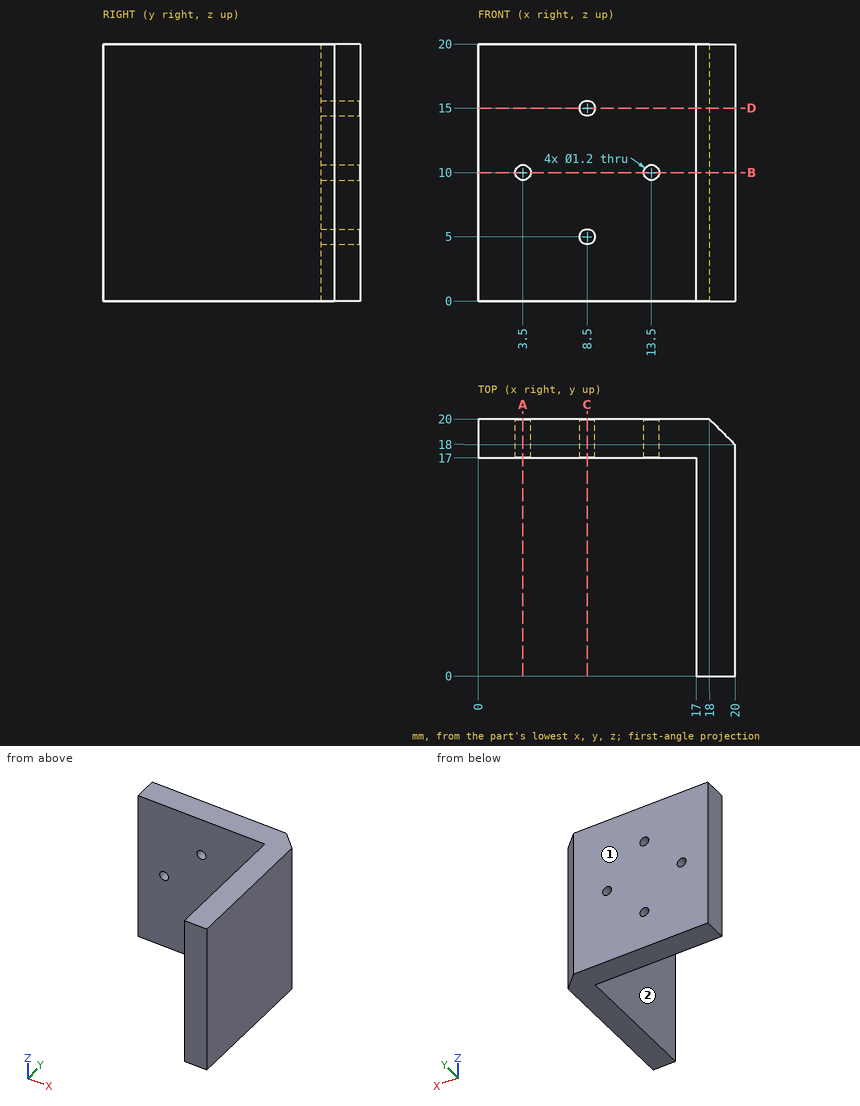
Study the drawing (mm; zero at the part's minimum x, y, z) and answer. A direction names the side the tool comes from. Round coordinates to 2 decimals unless told otherwise and drop trailing zeros. Write each loop counter-clockwise with the first axis right and the second up, starting at its lowest first coordinate (ties: lowest second). Pieces come first, ordered by that corner, then holes.
Q1. Find section B-B on z = 10. Determine the outline of the cut face in (x, y).
Values:
outline: (0, 17) - (2.9, 17) - (2.9, 20) - (0, 20) - close; (4.1, 17) - (12.9, 17) - (12.9, 20) - (4.1, 20) - close; (14.1, 17) - (17, 17) - (17, 0) - (20, 0) - (20, 18) - (18, 20) - (14.1, 20) - close
Q2. A tool of negligible diameter and unlimited length cuts with its end or side. For the marked faces 1 and 2, from which of +Z, -Z, +X, -X, +Y, -Y can it reach the whole face along a straight path? Write none if from no direction.
Values:
face 1: +Z, -Z, +X, -X, +Y
face 2: +Z, -Z, -X, -Y
Q3. Find section C-C on x = 8.5. Determine the outline of the cut face in (y, z).
Values:
outline: (17, 0) - (20, 0) - (20, 4.4) - (17, 4.4) - close; (17, 5.6) - (20, 5.6) - (20, 14.4) - (17, 14.4) - close; (17, 15.6) - (20, 15.6) - (20, 20) - (17, 20) - close
Q4. Flat-ended cylindrical pins translate along their axes: P1, Ø1.4, axis at x = 8.5, z = 15, coming from the -Y side; P2, Ø0.7, axis at x = 3.5, z = 10, coming from the -Y side; P3, Ø5, axis at y = 4.5, z = 5.5, coming from the -X side. Find the tip coordinate at first contact, or state that the pin passes through.
Values:
P1: stops at y = 17
P2: passes through
P3: stops at x = 17
Q5. Straight lines are drawn through the part: line 1 (Z direction, x = 13.5, y = 18.3); line 2 (X direction, y = 17.6, z = 5); line 3 (Y direction, x = 7.5, z = 12.75). For each, find the intervals that lie inside material, in ascending order.
Values:
line 1: z = 0 to 9.4, 10.6 to 20
line 2: x = 0 to 7.9, 9.1 to 20
line 3: y = 17 to 20
Q6. Find section A-A on x = 3.5. Determine the outline of the cut face in (y, z), and give its area (3 significant figures).
Values:
outline: (17, 0) - (20, 0) - (20, 9.4) - (17, 9.4) - close; (17, 10.6) - (20, 10.6) - (20, 20) - (17, 20) - close
area: 56.4 mm2
Q7. Find section D-D on z = 15. Determine the outline of the cut face in (x, y).
Values:
outline: (0, 17) - (7.9, 17) - (7.9, 20) - (0, 20) - close; (9.1, 17) - (17, 17) - (17, 0) - (20, 0) - (20, 18) - (18, 20) - (9.1, 20) - close
